from build123d import *

# Parameters (mm, degrees)
F1_DEPTH = 5
F2_DEPTH = 75
F3_DEPTH = 70


with BuildPart() as f1:
    # F0 (on Right) → F1 (new body)
    with BuildSketch(Plane.YZ):
        with BuildLine():
            Line((-11, -4), (-9.165151, -4))
            ThreePointArc((-9.165151, -4), (-10, 0), (-9.165151, 4))
            Line((-9.165151, 4), (-11, 4))
            Line((-11, 4), (-11, -4))
        make_face()
        with BuildLine():
            Line((-9.165151, -4), (9.165151, -4))
            ThreePointArc((9.165151, -4), (10, 0), (9.165151, 4))
            Line((9.165151, 4), (-9.165151, 4))
            ThreePointArc((-9.165151, 4), (-10, 0), (-9.165151, -4))
        make_face()
        with BuildLine():
            Line((9.165151, -4), (11, -4))
            Line((11, -4), (11, 4))
            Line((11, 4), (9.165151, 4))
            ThreePointArc((9.165151, 4), (10, 0), (9.165151, -4))
        make_face()
    extrude(amount=-F1_DEPTH)

    # F0 (on Right) → F2 (join)
    with BuildSketch(Plane.YZ):
        with BuildLine():
            Line((9.165151, -4), (11, -4))
            Line((11, -4), (11, 4))
            Line((11, 4), (9.165151, 4))
            ThreePointArc((9.165151, 4), (10, 0), (9.165151, -4))
        make_face()
        with BuildLine():
            Line((-9.165151, -4), (9.165151, -4))
            ThreePointArc((9.165151, -4), (10, 0), (9.165151, 4))
            Line((9.165151, 4), (-9.165151, 4))
            ThreePointArc((-9.165151, 4), (-10, 0), (-9.165151, -4))
        make_face()
        with BuildLine():
            Line((-11, -4), (-9.165151, -4))
            ThreePointArc((-9.165151, -4), (-10, 0), (-9.165151, 4))
            Line((-9.165151, 4), (-11, 4))
            Line((-11, 4), (-11, -4))
        make_face()
    extrude(amount=F2_DEPTH)

    # F0 (on Right) → F3 (cut)
    with BuildSketch(Plane.YZ):
        with BuildLine():
            Line((-9.165151, -4), (9.165151, -4))
            ThreePointArc((9.165151, -4), (10, 0), (9.165151, 4))
            Line((9.165151, 4), (-9.165151, 4))
            ThreePointArc((-9.165151, 4), (-10, 0), (-9.165151, -4))
        make_face()
    extrude(amount=F3_DEPTH, mode=Mode.SUBTRACT)


solid = f1.part
CAD build for the part. Positions are in the model's coordinates, mm. A direction names the side the tool comes from. Coordinates: 2 decimals unless noted, no trailing zeros. Loops run counter-clockwise (first coordinate to the right, second up) from the corner with the lowest first, then second, coordinate; pieces in that order, holes last. Notation, with made-up numbers: (-37, 39.25) - (5, 39.25) arc R14 ccw to (5, 62.25) - close; hole circle Ø5 at (38, 13). An arc over 180 degrees is marked (long way). Use one line per item in the form item = value. Start each with the question number.
1) Band-saw the part on C-C (z = -3). Give the cut face in (x, y), and give its area (3 significant figures).
2) Drill centre lines: L1, parallel to X at y = 5, z = -1.5; L2, parallel to Y at x = 49, z = -0.25; L3, parallel to Y at x = 3, z = -2.5. Where is each one in solid material? Low to high. Write a range as from..to.
3) Band-saw the part on D-D (z = 2.5). Give the cut face in (x, y).
4) Tool access for faces 1 (the face through (35, -10, -4)), 2 (the face through (35, 10, 0)): list every direction of +Z, -Z, +X, -X, +Y, -Y with a clear straight run to the whole face (end or side of a thin tool).
5) Flat gauge pin, fed straight in: pin 1 (1.5 mm diameter, centred on x = 36.5, y = 6.5, fed in from -Z). Where does the tip first touch, or does it go through?
6) Band-saw the part on B-B (x = 30.5). Give the cut face in (y, z).
7) Two-plate mould, pull along X, no slides. Class faces 3 (the face through (34, -11, 0)), 4 (the face through (-5, 0, 0)), 5 (the face through (0, 0, 0)): +X half, -X half, draft (parallel to the pull), parting line (faces both ways), or undercut.
8) Band-saw the part on A-A (y = -0.25). Give the cut face in (x, z).
Check values:
q1.outline = (-5, -11) - (75, -11) - (75, 11) - (-5, 11) - close; hole (0, -9.54) - (70, -9.54) - (70, 9.54) - (0, 9.54) - close
q1.area = 424 mm2
q2.L1 = -5..0, 70..75
q2.L2 = -11..-10, 10..11
q2.L3 = -11..-9.68, 9.68..11
q3.outline = (-5, -11) - (75, -11) - (75, 11) - (-5, 11) - close; hole (0, -9.68) - (70, -9.68) - (70, 9.68) - (0, 9.68) - close
q4.face_1 = -Z, +X, -X, +Y, -Y
q4.face_2 = none
q5.pin_1 = through
q6.outline = (-11, -4) - (-9.17, -4) arc R10 cw to (-9.17, 4) - (-11, 4) - close; (9.17, -4) - (11, -4) - (11, 4) - (9.17, 4) arc R10 cw to start
q7.face_3 = draft
q7.face_4 = -X half
q7.face_5 = undercut
q8.outline = (-5, -4) - (0, -4) - (0, 4) - (-5, 4) - close; (70, -4) - (75, -4) - (75, 4) - (70, 4) - close
